Read the model definition and answer for the solid it produces. Units are mm, in the model's axes. Face numbers are marked on the shaded views. A direction names the side the tool comes from. Give positions to 0.01 mm unless a question says otherwise; leave off trailing zeros. Write each loop counter-clockwise with the first axis right and the second up, starting at its lowest first coordinate (ties: lowest second). Pieces come first, ordered by that corner, then holes. Notation, with made-up numbers: (5, 66) -> (39, 66) arc R13 cw to (39, 89) -> close; hole circle Ø1 at (-7.75, 24). An arc over 180 degrees is marked (long way). Put each result on its own line as item: value. Start each with the question number.
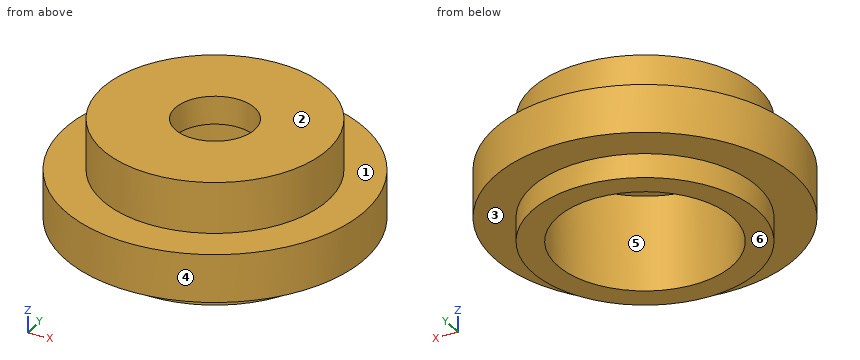
from build123d import *

# Parameters (mm, degrees)
F_3_8_CLEARANCE_HOLE1_D     = 10.0838
F_3_8_CLEARANCE_HOLE1_DEPTH = 15.621
SKETCH7_R                   = 11.1125
CUT_EXTRUDE2_DEPTH          = 12.065


with BuildPart() as part:
    # Sketch1 → Revolve1 (revolve)
    with BuildSketch(Plane(origin=(0, 0, 0), x_dir=(0, 0, -1), z_dir=(1, 0, 0))):
        Polygon((0, 0), (0, 14.2875), (6.477, 14.2875), (6.477, 19.05), (12.573, 19.05), (12.573, 14.2875), (15.621, 14.2875), (15.621, 0), align=None)
    revolve(axis=Axis((0, 0, 13.696708861), (0, 0, -1)))

    # 3/8 Clearance Hole1
    with Locations(Plane.XY):
        with Locations((0, 0)):
            Hole(F_3_8_CLEARANCE_HOLE1_D / 2, depth=F_3_8_CLEARANCE_HOLE1_DEPTH)

    # Sketch7 → Cut-Extrude2 (cut)
    with BuildSketch(Plane(origin=(0, 0, -15.621), x_dir=(-1, 0, 0), z_dir=(0, 0, -1))):
        Circle(SKETCH7_R)
    extrude(amount=-CUT_EXTRUDE2_DEPTH, mode=Mode.SUBTRACT)


solid = part.part
1) A cutting plane is placed at A-A on x = 0. Give the vertices of the cut face in (y, z).
2) Each of these flat-tipped pins is pushed along its axis until it touches: pin 1 Ø1.5 at (x, y) = (3.5, 4.5) entering from -Z; pin 2 Ø8 at (y, z) = (6.5, -2) entering from +X; pin 3 Ø1.5 at (y, z) = (-10, -4.5) entering from +X. Where does it stop, or does it pass through?
3) Straight lines are drawn through the part: line 1 (Y direction, x = -6.5, z = -7.75); line 2 (X direction, y = 1.5, z = -2); line 3 (Z direction, x = 6, y = 14). For each, find the intervals that lie inside material, in ascending order. Write a range as [from, to].
4) For a pull along Y with two mould halves and no side action, classify the marked faces 4, 5 and 6 as pulls with the +Y half, pulls with the -Y half, needs draft (parallel to the pull), parting line crosses it, or undercut.
5) For the marked faces 1, 2 and 3, determine the directions among +Z, -Z, +X, -X, +Y, -Y from which every point of the face is accessible in a straight line to the end or side of a thin tool.
6) A cutting plane is placed at D-D on y = 6.5. Give the vertices of the cut face in (x, z).
Results found:
1. outline: (-19.05, -12.57) -> (-14.29, -12.57) -> (-14.29, -15.62) -> (-11.11, -15.62) -> (-11.11, -3.56) -> (-5.04, -3.56) -> (-5.04, 0) -> (-14.29, 0) -> (-14.29, -6.48) -> (-19.05, -6.48) -> close; (5.04, -3.56) -> (11.11, -3.56) -> (11.11, -15.62) -> (14.29, -15.62) -> (14.29, -12.57) -> (19.05, -12.57) -> (19.05, -6.48) -> (14.29, -6.48) -> (14.29, 0) -> (5.04, 0) -> close
2. pin 1: stops at z = -3.56
2. pin 2: stops at x = 14.07
2. pin 3: stops at x = 10.89
3. line 1: y = [-17.91, -9.01], [9.01, 17.91]
3. line 2: x = [-14.21, -4.81], [4.81, 14.21]
3. line 3: z = [-12.57, -6.48]
4. face 4: parting line crosses it
4. face 5: undercut
4. face 6: needs draft
5. face 1: +Z
5. face 2: +Z, +X, -X, +Y, -Y
5. face 3: -Z
6. outline: (-17.91, -12.57) -> (-12.72, -12.57) -> (-12.72, -15.62) -> (-9.01, -15.62) -> (-9.01, -3.56) -> (9.01, -3.56) -> (9.01, -15.62) -> (12.72, -15.62) -> (12.72, -12.57) -> (17.91, -12.57) -> (17.91, -6.48) -> (12.72, -6.48) -> (12.72, 0) -> (-12.72, 0) -> (-12.72, -6.48) -> (-17.91, -6.48) -> close
